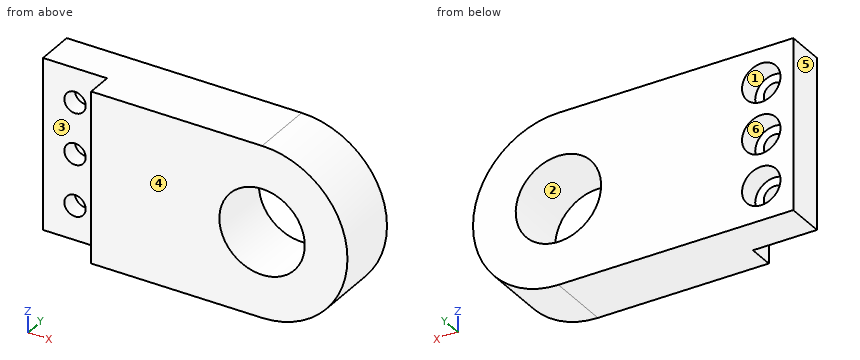
```python
from build123d import *

# Parameters (mm, degrees)
SKETCH_1_R          = 10
EXTRUDE_1_DEPTH     = 15
SKETCH_2_W          = 15
SKETCH_2_H          = 9
EXTRUDE_2_DEPTH     = 40
CUT_EXTRUDE_1_REACH = 62.415
SKETCH_3_R          = 2.5
SKETCH_3_3_R        = 4.5
SKETCH_3_3_R_2      = 2.5
CUT_EXTRUDE_2_DEPTH = 5


with BuildPart() as part:
    # 草图1 → 凸台-拉伸1 (new body)
    with BuildSketch(Plane(origin=(0, 0, 0), x_dir=(1, 0, 0), z_dir=(0, 1, 0))):
        with BuildLine():
            Line((0, 20), (-40, 20))
            Line((-40, 20), (-40, -20))
            Line((-40, -20), (0, -20))
            ThreePointArc((0, -20), (20, 0), (0, 20))
        make_face()
        with Locations(Location((0, 0, 0), (0, 0, 270))):
            Circle(SKETCH_1_R, mode=Mode.SUBTRACT)
    extrude(amount=EXTRUDE_1_DEPTH)

    # 草图2 → 凸台-拉伸2 (add)
    with BuildSketch(Plane.XY.offset(20)):
        with Locations((-47.5, 10.5)):
            Rectangle(SKETCH_2_W, SKETCH_2_H)
    extrude(amount=-EXTRUDE_2_DEPTH)

    # 草图3 → 切除-拉伸1 (cut, up to next)
    with BuildSketch(Plane(origin=(0, 15, 0), x_dir=(1, 0, 0), z_dir=(0, 1, 0)), mode=Mode.PRIVATE) as cut_extrude_1_sk1:
        with Locations(Location((-47.5, 12, 0), (0, 0, 270))):
            Circle(SKETCH_3_R)
    cut_extrude_1_tool1 = extrude(cut_extrude_1_sk1.sketch, amount=-CUT_EXTRUDE_1_REACH, mode=Mode.PRIVATE) & part.part
    # 草图3 → 切除-拉伸1 (cut, up to next)
    with BuildSketch(Plane(origin=(0, 15, 0), x_dir=(1, 0, 0), z_dir=(0, 1, 0)), mode=Mode.PRIVATE) as cut_extrude_1_sk2:
        with Locations(Location((-47.5, 0, 0), (0, 0, 270))):
            Circle(SKETCH_3_R)
    cut_extrude_1_tool2 = extrude(cut_extrude_1_sk2.sketch, amount=-CUT_EXTRUDE_1_REACH, mode=Mode.PRIVATE) & part.part
    # 草图3 → 切除-拉伸1 (cut, up to next)
    with BuildSketch(Plane(origin=(0, 15, 0), x_dir=(1, 0, 0), z_dir=(0, 1, 0)), mode=Mode.PRIVATE) as cut_extrude_1_sk3:
        with Locations(Location((-47.5, -12, 0), (0, 0, 270))):
            Circle(SKETCH_3_R)
    cut_extrude_1_tool3 = extrude(cut_extrude_1_sk3.sketch, amount=-CUT_EXTRUDE_1_REACH, mode=Mode.PRIVATE) & part.part
    add(cut_extrude_1_tool1.solids().sort_by_distance((-47.5, 15, -12))[0], mode=Mode.SUBTRACT)
    add(cut_extrude_1_tool2.solids().sort_by_distance((-47.5, 15, 0))[0], mode=Mode.SUBTRACT)
    add(cut_extrude_1_tool3.solids().sort_by_distance((-47.5, 15, 12))[0], mode=Mode.SUBTRACT)

    # 草图3<3> → 切除-拉伸2 (cut)
    # profile 1 of 3: a face of its own
    with BuildSketch(Plane(origin=(0, 15, 0), x_dir=(1, 0, 0), z_dir=(0, 1, 0))):
        with Locations(Location((-47.5, 12, 0), (0, 0, 270))):
            Circle(SKETCH_3_3_R)
        with Locations(Location((-47.5, 12, 0), (0, 0, 270))):
            Circle(SKETCH_3_3_R_2, mode=Mode.SUBTRACT)
    # profile 2 of 3: a face of its own
    with BuildSketch(Plane(origin=(0, 15, 0), x_dir=(1, 0, 0), z_dir=(0, 1, 0))):
        with Locations(Location((-47.5, 0, 0), (0, 0, 270))):
            Circle(SKETCH_3_3_R)
        with Locations(Location((-47.5, 0, 0), (0, 0, 270))):
            Circle(SKETCH_3_3_R_2, mode=Mode.SUBTRACT)
    # profile 3 of 3: a face of its own
    with BuildSketch(Plane(origin=(0, 15, 0), x_dir=(1, 0, 0), z_dir=(0, 1, 0))):
        with Locations(Location((-47.5, -12, 0), (0, 0, 270))):
            Circle(SKETCH_3_3_R)
        with Locations(Location((-47.5, -12, 0), (0, 0, 270))):
            Circle(SKETCH_3_3_R_2, mode=Mode.SUBTRACT)
    extrude(amount=-CUT_EXTRUDE_2_DEPTH, mode=Mode.SUBTRACT)


solid = part.part
```
Work out the finished part from the listing and answer in its coordinate system (mm). Face numbers are marked on the shaded views. A direction names the side the tool comes from. Give positions to 0.01 mm unless a question says otherwise; leave off trailing zeros. Order: outer loops, then holes, each group sorted by start corner. A loop starts at its lowest first (then second) coordinate and runs counter-clockwise, first axis right, second up. Notation, with made-up numbers: (56.5, 57) -> (92.5, 57) arc R14 ccw to (92.5, 82) -> close; hole circle Ø4 at (22, 55.25). An arc over 180 degrees is marked (long way). Answer as CSV lines item,"result". Start each with the question number.
(1) For a pull along X with two mould halves and no side action, classify the marked faces 4, 5 and 6 as released by +X, released by -X, zero draft, split by the parting line, or undercut.
(2) Which of the six approach directions +Z, -Z, +X, -X, +Y, -Y give full straight-line access (tool end or side, diameter ignored) to the marked faces 1, 2 and 3?
(3) Section C-C, the plane x = -8 is taken. Write down the section's boundary in (y, z).
(4) Consider line 1 along X through (y, z) = (14, 15); line 2 along Z through (x, y) = (-44, 11.5); line 3 along X through (y, z) = (11, -1). Determine where each line is inside the solid, lowest interval first.
(5) Section D-D, the plane z = 12 is taken. Write down the section's boundary in (x, y), plus the area to 3 significant figures.
(6) Each of these flat-tipped pins is pushed along its axis until it touches: pin 1 Ø4.5 at (x, z) = (-47.5, 0) entering from +Y; pin 2 Ø5.5 at (x, z) = (-47.5, -12) entering from +Y; pin 3 Ø16.5 at (x, z) = (-49.5, 7) entering from -Y; pin 4 Ø6.5 at (y, z) = (2, 4.5) entering from -X. Where does it stop, or does it pass through?
(7) Section B-B, the plane x = -47.5 is taken. Write down the section's boundary in (y, z), plus the area to 3 significant figures.
(8) Section A-A, the plane z = 0 is taken. Write down the section's boundary in (x, y).
Entries:
1,face 4,"zero draft"
1,face 5,"released by -X"
1,face 6,"undercut"
2,face 1,"+Y"
2,face 2,"+Y, -Y"
2,face 3,"+Z, -Z, -X, -Y"
3,outline,"(0, -20) -> (15, -20) -> (15, -6) -> (0, -6) -> close; (0, 6) -> (15, 6) -> (15, 20) -> (0, 20) -> close"
4,line 1,"-55 to -50.85, -44.15 to 13.23"
4,line 2,"-20 to -14.83, -9.17 to -2.83, 2.83 to 9.17, 14.83 to 20"
4,line 3,"-55 to -51.89, -43.11 to -9.95, 9.95 to 19.97"
5,outline,"(-55, 6) -> (-50, 6) -> (-50, 10) -> (-52, 10) -> (-52, 15) -> (-55, 15) -> close; (-45, 6) -> (-40, 6) -> (-40, 0) -> (16, 0) -> (16, 15) -> (-43, 15) -> (-43, 10) -> (-45, 10) -> close"
5,area,"910 mm²"
6,pin 1,"through"
6,pin 2,"y = 10"
6,pin 3,"y = 6"
6,pin 4,"x = -40"
7,outline,"(6, -20) -> (15, -20) -> (15, -16.5) -> (10, -16.5) -> (10, -14.5) -> (6, -14.5) -> close; (6, -9.5) -> (10, -9.5) -> (10, -7.5) -> (15, -7.5) -> (15, -4.5) -> (10, -4.5) -> (10, -2.5) -> (6, -2.5) -> close; (6, 2.5) -> (10, 2.5) -> (10, 4.5) -> (15, 4.5) -> (15, 7.5) -> (10, 7.5) -> (10, 9.5) -> (6, 9.5) -> close; (6, 14.5) -> (10, 14.5) -> (10, 16.5) -> (15, 16.5) -> (15, 20) -> (6, 20) -> close"
7,area,"165 mm²"
8,outline,"(-55, 6) -> (-50, 6) -> (-50, 10) -> (-52, 10) -> (-52, 15) -> (-55, 15) -> close; (-45, 6) -> (-40, 6) -> (-40, 0) -> (-10, 0) -> (-10, 15) -> (-43, 15) -> (-43, 10) -> (-45, 10) -> close; (10, 0) -> (20, 0) -> (20, 15) -> (10, 15) -> close"
